Work out the finished part from the listing and answer in its coordinate system (mm). A direction names the side the tool comes from. Give positions to 0.01 mm unless a question says otherwise; leave off trailing zeros. Loops run counter-clockwise (first coordinate to the right, second up) from the corner with the lowest first, then second, coordinate; pieces in that order, holes last.
```python
from build123d import *

# Parameters (mm, degrees)
EXTRUDE_1_DEPTH      = 100
EXTRUDE_1_DEPTH_BACK = 150


with BuildPart() as part:
    # Эскиз1 → Бобышка-Вытянуть1 (new, two sides: drawn at the far end of the back side and taken through both)
    with BuildSketch(Plane(origin=(0, 0, 0), x_dir=(1, 0, 0), z_dir=(0, 1, 0)).offset(-EXTRUDE_1_DEPTH_BACK)):
        with BuildLine():
            Line((-56, 0), (-4, 0))
            ThreePointArc((-4, 0), (-1.171572875, -1.171572875), (0, -4))
            Line((0, -4), (0, -56))
            ThreePointArc((0, -56), (-1.171572875, -58.828427125), (-4, -60))
            Line((-4, -60), (-56, -60))
            ThreePointArc((-56, -60), (-58.828427125, -58.828427125), (-60, -56))
            Line((-60, -56), (-60, -4))
            ThreePointArc((-60, -4), (-58.828427125, -1.171572875), (-56, 0))
        make_face()
        with BuildLine():
            Line((-53, -4), (-7, -4))
            ThreePointArc((-7, -4), (-4.878679656, -4.878679656), (-4, -7))
            Line((-4, -7), (-4, -53))
            ThreePointArc((-4, -53), (-4.878679656, -55.121320344), (-7, -56))
            Line((-7, -56), (-53, -56))
            ThreePointArc((-53, -56), (-55.121320344, -55.121320344), (-56, -53))
            Line((-56, -53), (-56, -7))
            ThreePointArc((-56, -7), (-55.121320344, -4.878679656), (-53, -4))
        make_face(mode=Mode.SUBTRACT)
    extrude(amount=EXTRUDE_1_DEPTH + EXTRUDE_1_DEPTH_BACK)


solid = part.part
```
Q1. Section B-B on x = -29 is taken. Give the vertices of the cut face in (y, z), plus the area to 3 significant figures.
Q2. Section C-C on y = -34 is taken. Give the vertices of the cut face in (x, z), plus the area to 3 significant figures.
Q3. Section A-A on z = 21 is taken. Give the vertices of the cut face in (x, y).
Q4. Determine the mould class of faces 1 (the face through (-1.141, -26.75, 58.797)), 2 (the face through (-56.2, 100, 29.6)), 3 (the face through (-30, -27, 56)) for opening direction Z: +Z half, -Z half, draft (parallel to the pull), parting line (faces both ways), or undercut.
Q5. Consider line 1 along Z through (x, y) = (-19, -65); line 2 along X through (y, z) = (50.5, 37.5); line 3 along X through (y, z) = (-38.5, 54). Determine where each line is inside the solid, lowest interval first.
Q6. Which of the six approach directions +Z, -Z, +X, -X, +Y, -Y give full straight-line access (tool end or side, diameter ignored) to faces 4 (the face through (-58.797, -26.75, 58.859)), 5 (the face through (-56, -27, 30))?
Check result:
1. outline: (-150, 0) - (100, 0) - (100, 4) - (-150, 4) - close; (-150, 56) - (100, 56) - (100, 60) - (-150, 60) - close
1. area: 2,000 mm2
2. outline: (-60, 4) arc R4 ccw to (-56, 0) - (-4, 0) arc R4 ccw to (0, 4) - (0, 56) arc R4 ccw to (-4, 60) - (-56, 60) arc R4 ccw to (-60, 56) - close; hole (-56, 7) arc R3 ccw to (-53, 4) - (-7, 4) arc R3 ccw to (-4, 7) - (-4, 53) arc R3 ccw to (-7, 56) - (-53, 56) arc R3 ccw to (-56, 53) - close
2. area: 890 mm2
3. outline: (-60, -150) - (-56, -150) - (-56, 100) - (-60, 100) - close; (-4, -150) - (0, -150) - (0, 100) - (-4, 100) - close
4. face 1: +Z half
4. face 2: draft
4. face 3: undercut
5. line 1: z = 0 to 4, 56 to 60
5. line 2: x = -60 to -56, -4 to 0
5. line 3: x = -60 to -55.83, -4.17 to 0
6. face 4: +Z, -X, +Y, -Y
6. face 5: +Y, -Y
